from build123d import *

# Parameters (mm, degrees)
F1_DEPTH = 5
F2_DEPTH = 1


with BuildPart() as f1:
    # F0 (on Top) → F1 (new body)
    with BuildSketch(Plane.XY):
        Polygon((19.19481, 70.408), (17.181838, 73.022946), (7.964966, 73.022946), (-20.01172, 73.433359), (-21.430185, 70.408), (-31.604451, 70.408), (-35.205591, 70.408), (-35.205591, -4), (26.194409, -4), (26.194409, 70.408), align=None)
        Polygon((22.194409, 0), (-31.205591, 0), (-31.205591, 66.408), (-18.887785, 66.408), (-17.486888, 69.39589), (7.935628, 69.022946), (15.213112, 69.022946), (17.226085, 66.408), (22.194409, 66.408), align=None, mode=Mode.SUBTRACT)
    extrude(amount=F1_DEPTH)

    # F0 (on Top) → F2 (join)
    with BuildSketch(Plane.XY):
        Polygon((-31.205591, 66.408), (-31.205591, 0), (22.194409, 0), (22.194409, 66.408), (17.226085, 66.408), (15.213112, 69.022946), (7.935628, 69.022946), (-17.486888, 69.39589), (-18.887785, 66.408), align=None)
    extrude(amount=F2_DEPTH)


solid = f1.part
Here's how the part is built. I have some questions about the finished solid (model axes, mm). A direction names the side the tool comes from. Coordinates: 2 decimals unless noted, no trailing zeros. Loops run counter-clockwise (first coordinate to the right, second up) from the corner with the lowest first, then second, coordinate; pieces in that order, holes last. Notation, with made-up numbers: (-32, 76) -> (3, 76) arc R14 ccw to (3, 84) -> close; hole circle Ø2 at (29.25, 86). An arc over 180 degrees is marked (long way). Use one line per item in the form item = value. Start each with the question number.
(1) If we section it at B-B (x = 20.5): Please give me the cut outline in (y, z).
(2) Will these pins go through, and if not, where does the flat tip stop? pin 1 (1.5 mm diameter, centred on x = -31.5, z = 3.5, fed in from +Y); pin 2 (1.2 mm diameter, centred on x = 5, z = 2.5, fed in from +Y); pin 3 (1 mm diameter, centred on x = -12, z = 3.5, fed in from +Y).
(3) If we section it at A-A (z = 3.85): Please give me the cut outline in (x, y).
(4) If we section it at C-C (y = 65.5): Please give me the cut outline in (x, z).
(5) Please list where these lines run through material, in increasing order: line 1 along X through (y, z) = (22, 1.7); line 2 along Y through (x, z) = (-22.5, 3.15); line 3 along Y through (x, z) = (12, 3.7).
(6) We'd pull the mould along Y, two halves only. Please class faces 1 (the face through (-5, 35, 0)), 2 (the face through (-20.71, 71.94, 2.46)), 3 (the face through (20, 66.408, 3)): pulls with the +Y half, pulls with the -Y half, needs draft (parallel to the pull), parting line crosses it, or undercut.
(7) On a 3-axis mill with a long thin cutter (end or side, diameter ignored), from which of +Z, -Z, +X, -X, +Y, -Y can I reach the whole of each face in a straight line? I mean faces 4 (the face through (-25, 66.408, 3)), 5 (the face through (-28, 70.408, 2)), 6 (the face through (23, 70.408, 2)). Say none if no direction works.
Verdict:
q1.outline = (-4, 0) -> (70.41, 0) -> (70.41, 5) -> (66.41, 5) -> (66.41, 1) -> (0, 1) -> (0, 5) -> (-4, 5) -> close
q2.pin_1 = 70.41
q2.pin_2 = 73.08
q2.pin_3 = 73.32
q3.outline = (-35.21, -4) -> (26.19, -4) -> (26.19, 70.41) -> (19.19, 70.41) -> (17.18, 73.02) -> (7.96, 73.02) -> (-20.01, 73.43) -> (-21.43, 70.41) -> (-35.21, 70.41) -> close; hole (-31.21, 0) -> (22.19, 0) -> (22.19, 66.41) -> (17.23, 66.41) -> (15.21, 69.02) -> (7.94, 69.02) -> (-17.49, 69.4) -> (-18.89, 66.41) -> (-31.21, 66.41) -> close
q4.outline = (-35.21, 0) -> (26.19, 0) -> (26.19, 5) -> (22.19, 5) -> (22.19, 1) -> (-31.21, 1) -> (-31.21, 5) -> (-35.21, 5) -> close
q5.line_1 = -35.21 to -31.21, 22.19 to 26.19
q5.line_2 = -4 to 0, 66.41 to 70.41
q5.line_3 = -4 to 0, 69.02 to 73.02
q6.face_1 = needs draft
q6.face_2 = pulls with the +Y half
q6.face_3 = undercut
q7.face_4 = +Z
q7.face_5 = +Z, -Z, -X, +Y
q7.face_6 = +Z, -Z, +X, +Y
